Geometry: final body of the model. Coordinates: model frame, mm. Give positions to 0.01 mm unless a question says otherwise; leave off trailing zeros. Order: outer loops, then holes, each group sorted by start corner. A loop starts at its lowest first (then second) coordinate and runs counter-clockwise, first axis right, second up. Notation, with made-up numbers: (-25, 44.25) -> (-9, 44.25) arc R27 cw to (-9, 61.25) -> close; hole circle Ø7 at (49, 5.5). An arc over 180 degrees is marked (long way). One line per question, with ' | ' between items. Start each with the question number.
(1) Section D-D (x = 10.5). Return loops of the section in (y, z) (3 decimals), then the cut area to 3 significant figures.
(2) Section A-A (x = 0). Return loops of the section in (y, z) (3 decimals), then the cut area to 3 significant figures.
(3) First-contact query: pin 1 Ø1 at (y, z) = (1.5, 2) entering from +X; pin 2 Ø1.6 at (y, z) = (1, 1) entering from -X; pin 3 Ø1.5 at (y, z) = (26, 0.5) entering from -X. Flat tips, straight axial feed; report the tip coordinate or a pass-through.
(4) Section C-C (y = 29). Return loops of the section in (x, z) (1 decimal).
(5) Ray query, L1, parallel to Y at x = 0, z = 0.9; L2, parallel to Y at x = -10.5, z = 1.7 (3 decimals); L3, parallel to X at y = 2.5, z = 2.9. Return the intervals inside material, ascending.
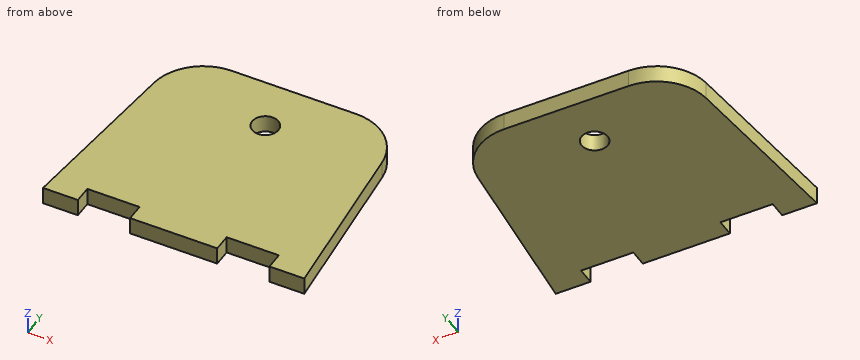
```python
from build123d import *

# Parameters (mm, degrees)
SKETCH1_R           = 2.38125
BOSS_EXTRUDE1_DEPTH = 3.175
SKETCH2_W           = 9.525
SKETCH2_H           = 3.175
CUT_EXTRUDE1_DEPTH  = 47.881796705


with BuildPart() as part:
    # Sketch1 → Boss-Extrude1 (new body)
    with BuildSketch(Plane.XY):
        with BuildLine():
            Line((-11.330339119, 40.259), (11.330339119, 40.259))
            ThreePointArc((11.330339119, 40.259), (17.739736735, 37.779938348), (20.812800106, 31.633198887))
            Line((20.812800106, 31.633198887), (23.8125, 0))
            Line((23.8125, 0), (-23.8125, 0))
            Line((-23.8125, 0), (-20.812800106, 31.633198887))
            ThreePointArc((-20.812800106, 31.633198887), (-17.739736735, 37.779938348), (-11.330339119, 40.259))
        make_face()
        with Locations((0, 30.734)):
            Circle(SKETCH1_R, mode=Mode.SUBTRACT)
    extrude(amount=BOSS_EXTRUDE1_DEPTH)

    # Sketch2 → Cut-Extrude1 (cut, through all)
    with BuildSketch(Plane.XY.offset(3.175)):
        with Locations((-12.7, 1.5875)):
            Rectangle(SKETCH2_W, SKETCH2_H)
        with Locations((12.7, 1.5875)):
            Rectangle(SKETCH2_W, SKETCH2_H)
    extrude(amount=-CUT_EXTRUDE1_DEPTH, mode=Mode.SUBTRACT)


solid = part.part
```
Response:
1) outline: (3.175, 0) -> (40.259, 0) -> (40.259, 3.175) -> (3.175, 3.175) -> close | area: 118 mm^2
2) outline: (0, 0) -> (28.353, 0) -> (28.353, 3.175) -> (0, 3.175) -> close; (33.115, 0) -> (40.259, 0) -> (40.259, 3.175) -> (33.115, 3.175) -> close | area: 113 mm^2
3) pin 1: stops at x = 23.72 | pin 2: stops at x = -23.79 | pin 3: stops at x = -21.42
4) outline: (-21.1, 0) -> (-1.6, 0) -> (-1.6, 3.2) -> (-21.1, 3.2) -> close; (1.6, 0) -> (21.1, 0) -> (21.1, 3.2) -> (1.6, 3.2) -> close
5) L1: y = 0 to 28.35, 33.12 to 40.26 | L2: y = 3.175 to 40.259 | L3: x = -23.58 to -17.46, -7.94 to 7.94, 17.46 to 23.58
